Check sheet for the modelled part. Datum: model origin and axes. Units: mm. A direction names the side the tool comes from. Give positions to 0.01 mm unless a question says otherwise; leave off trailing zeros. Write each loop counter-clockwise with the first axis right and the second up, starting at its lowest first coordinate (ties: lowest second). Pieces come first, ordered by that corner, then holes. Notation, with made-up numbers: (61.5, 10.5) -> (76.5, 10.5) arc R12 ccw to (76.5, 19.5) -> close; hole circle Ø11 at (25.25, 43.5). An arc over 180 degrees is marked (long way). Use a Markdown table: item, result. Add a question column.
1. Cross-section at A-A (x = -1.5). Enter the section's corners in (y, z).
2. Gauge pin test, flat ends, axial feed: P1, Ø8, axis at y = -20, z = 5.5, coming from the +X side; P2, Ø2, axis at x = 20, z = 5, coming from the +Y side; P3, Ø1, axis at x = 20, z = 13.5, coming from the -Y side. Record the tip position at first contact, or that the pin passes through.
3. Cross-section at D-D (x = 27). Enter the section's corners in (y, z), then the cut area to 3 significant figures.
4. Scan lines: probe 1 along X at (y, z) = (0, 10.5); probe 2 along X at (y, z) = (-36, 6.25); probe 3 along Y at (x, z) = (-1, 2.75). Record each from-to range of solid material in increasing order. Write a range as [from, to].
5. Cross-section at B-B (y = -57). Enter the section's corners in (x, z), then the cut area to 3 significant figures.
6. Set-up check for faces 4 (the flat face through (-0.4, -12, 8)), 5 (the flat face through (10, -41, 16)), 6 (the cylindrical face through (6.26, -15.1, 7.89)): record each of +Z, -Z, +X, -X, +Y, -Y from which the full face is reachable in a straight line by a thin tool's end or side.
7. Cross-section at C-C (y = -70). Enter the section's corners in (x, z).
8. Release check for a two-part mould opening along X. For faces 1 (the flat face through (-15, -44, 8)), 2 (the cylindrical face through (4.565, -10.23, 7.888)), 3 (the flat face through (10, -41, 0)) record: released by +X, released by -X, zero draft, split by the parting line, or undercut.
from build123d import *

# Parameters (mm, degrees)
PAD_DEPTH = 16


with BuildPart() as part:
    # Sketch008 → Pad (new body)
    with BuildSketch(Plane.XY):
        with BuildLine():
            Line((-15, -36.103415), (-13.488123, 0.576563))
            ThreePointArc((-9.888981, 9.384513), (-12.459776, 5.295679), (-13.488123, 0.576563))
            ThreePointArc((-7.476837, 9.129029), (-8.617886, 9.870686), (-9.888981, 9.384513))
            Line((-7.476837, 9.129029), (-6.901924, 8.13325))
            ThreePointArc((-7, 4.974937), (-6.501445, 6.540134), (-6.901924, 8.13325))
            ThreePointArc((-7, 4.974937), (-8.464339, -0.800395), (-6, -6.22495))
            ThreePointArc((-5.166667, -8.299933), (-5.382784, -7.181899), (-6, -6.22495))
            Line((-5.166667, -8.299933), (-5.166667, -8.799933))
            ThreePointArc((-5.166667, -8.799933), (-4.58088, -10.214147), (-3.166667, -10.799933))
            Line((-3.166667, -10.799933), (-0.4, -10.799933))
            Line((-0.4, -10.799933), (-0.4, -13.799933))
            Line((-3.166667, -13.799933), (-0.4, -13.799933))
            ThreePointArc((-3.166667, -13.799933), (-6.230796, -15.069137), (-7.5, -18.133266))
            Line((-7.5, -18.133266), (-7.5, -46.090027))
            ThreePointArc((-7.5, -46.090027), (-6.390434, -50.668257), (-3.307962, -54.230517))
            Line((-3.307962, -54.230517), (3.108659, -58.808557))
            ThreePointArc((3.108659, -58.808557), (9.457708, -58.836624), (11.602837, -52.860869))
            Line((8.136694, -40.367919), (11.602837, -52.860869))
            ThreePointArc((7.5, -35.691584), (7.659904, -38.051324), (8.136694, -40.367919))
            Line((7.5, -35.691584), (7.5, -18.133266))
            ThreePointArc((7.5, -18.133266), (6.230796, -15.069137), (3.166667, -13.799933))
            Line((0.4, -13.799933), (3.166667, -13.799933))
            Line((0.4, -10.799933), (0.4, -13.799933))
            Line((0.4, -10.799933), (3.166667, -10.799933))
            ThreePointArc((3.166667, -10.799933), (4.58088, -10.214147), (5.166667, -8.799933))
            Line((5.166667, -8.299933), (5.166667, -8.799933))
            ThreePointArc((6, -6.22495), (5.382784, -7.181899), (5.166667, -8.299933))
            ThreePointArc((6, -6.22495), (8.464339, -0.800395), (7, 4.974937))
            ThreePointArc((6.901924, 8.13325), (6.501445, 6.540134), (7, 4.974937))
            Line((7.476837, 9.129029), (6.901924, 8.13325))
            ThreePointArc((9.888981, 9.384513), (8.617886, 9.870686), (7.476837, 9.129029))
            ThreePointArc((13.488123, 0.576563), (12.459776, 5.295679), (9.888981, 9.384513))
            Line((15, -36.103415), (13.488123, 0.576563))
            ThreePointArc((15, -36.103415), (15.518303, -38.894431), (16.799996, -41.427348))
            Line((35.043138, -67.481255), (16.799996, -41.427348))
            ThreePointArc((35.043138, -67.481255), (21.967147, -79.759147), (10.666391, -93.688291))
            Line((10.666391, -93.688291), (-12.287281, -60.90705))
            ThreePointArc((-15, -52.303404), (-14.305754, -56.813991), (-12.287281, -60.90705))
            Line((-15, -36.103415), (-15, -52.303404))
        make_face()
    extrude(amount=PAD_DEPTH)


solid = part.part
Worked answers:
| question | item | result |
|---|---|---|
| 1 | outline | (-76.31, 0) -> (-55.52, 0) -> (-55.52, 16) -> (-76.31, 16) -> close; (-13.8, 0) -> (-10.8, 0) -> (-10.8, 16) -> (-13.8, 16) -> close |
| 2 | P1 | stops at x = 14.5 |
| 2 | P2 | stops at y = -44.57 |
| 2 | P3 | stops at y = -82.49 |
| 3 | outline | (-74.63, 0) -> (-55.99, 0) -> (-55.99, 16) -> (-74.63, 16) -> close |
| 3 | area | 298 mm² |
| 4 | probe 1 | x = [-13.51, -8.5], [8.5, 13.51] |
| 4 | probe 2 | x = [-15, -7.5], [7.5, 15] |
| 4 | probe 3 | y = [-77.03, -55.88], [-13.8, -10.8] |
| 5 | outline | (-14.25, 0) -> (0.57, 0) -> (0.57, 16) -> (-14.25, 16) -> close; (11.11, 0) -> (27.7, 0) -> (27.7, 16) -> (11.11, 16) -> close |
| 5 | area | 503 mm² |
| 6 | face 4 | +Z, -Z, +Y |
| 6 | face 5 | +Z, +X, -X, +Y, -Y |
| 6 | face 6 | +Z, -Z |
| 7 | outline | (-5.92, 0) -> (32.06, 0) -> (32.06, 16) -> (-5.92, 16) -> close |
| 8 | face 1 | released by -X |
| 8 | face 2 | undercut |
| 8 | face 3 | zero draft |
